Part model, mm, in its own coordinate system. A direction names the side the tool comes from. Coordinates: 2 decimals unless noted, no trailing zeros. Loops run counter-clockwise (first coordinate to the right, second up) from the corner with the lowest first, then second, coordinate; pieces in that order, holes last. Notation, with made-up numbers: M -34.75,80.5 L -19.75,80.5 A20 ccw -19.75,107.5 Z; hole C 88.25,39.5 d11. An arc over 180 degrees is marked long. Answer as CSV lines item,"result". Start each with the question number.
from build123d import *

# Parameters (mm, degrees)
SKETCH_W     = 30
SKETCH_H     = 30
PAD_DEPTH    = 2
SKETCH001_W  = 25
SKETCH001_H  = 25
PAD001_DEPTH = 1.5
FILLET_R     = 3


with BuildPart() as part:
    # Sketch → Pad (new body)
    with BuildSketch(Plane.XY):
        with Locations((-15, 15)):
            Rectangle(SKETCH_W, SKETCH_H)
    extrude(amount=PAD_DEPTH)

    # Sketch001 (on Face6 of Pad) → Pad001 (join)
    with BuildSketch(Plane.XY.offset(2)):
        with Locations((-15, 15)):
            Rectangle(SKETCH001_W, SKETCH001_H)
    extrude(amount=PAD001_DEPTH)

    # Fillet
    fillet_edges = [part.edges().sort_by_distance(p)[0] for p in [
        (-30, 0, 1),
        (0, 0, 1),
        (0, 30, 1),
        (-30, 30, 1),
    ]]
    fillet(fillet_edges, radius=FILLET_R)


solid = part.part
Q1. Tool access for faces 1 (the face through (-15, 27.5, 3)), 2 (the face through (-2.5, 15, 3)), 3 (the face through (-27.5, 15, 3)): list every direction of +Z, -Z, +X, -X, +Y, -Y with a clear straight run to the whole face (end or side of a thin tool).
Q2. Flat gauge pins, fed straight in: P1, Ø10, axis at x = -4, y = 7, coming from the -Z side; P2, Ø0.8, axis at x = -13.5, z = 3, coming from the -Y side. Where does each tip first touch, or does it go through?
Q3. Wall check: L1, parallel to X at y = 9.25, z = 2.75; L2, parallel to Z at x = -1.75, y = 23; L3, parallel to Y at x = -21, z = 2.1. Give the ranges that are in metal, low to high.
Q4. Slice it at B-B, the plane y = 14.75. Write the cut outline in (x, z), and give its area (3 significant figures).
Q5. Slice it at A-A, the plane x = -23.75. Write the cut outline in (y, z).
Solved:
1,face 1,"+Z, +X, -X, +Y"
1,face 2,"+Z, +X, +Y, -Y"
1,face 3,"+Z, -X, +Y, -Y"
2,P1,"stops at z = 0"
2,P2,"stops at y = 2.5"
3,L1,"x = -27.5 to -2.5"
3,L2,"z = 0 to 2"
3,L3,"y = 2.5 to 27.5"
4,outline,"M -30,0 L 0,0 L 0,2 L -2.5,2 L -2.5,3.5 L -27.5,3.5 L -27.5,2 L -30,2 Z"
4,area,"97.5 mm2"
5,outline,"M 0,0 L 30,0 L 30,2 L 27.5,2 L 27.5,3.5 L 2.5,3.5 L 2.5,2 L 0,2 Z"
